Geometry check sheet. Reference: the model listing, model coordinates, mm. A direction names the side the tool comes from. Coordinates: 2 decimals unless noted, no trailing zeros. Write each loop counter-clockwise with the first axis right and the second up, starting at its lowest first coordinate (ties: lowest second). Pieces come first, ordered by that corner, then holes. Notation, with made-up numbers: (-5.5, 80.5) -> (52.5, 80.5) arc R15 cw to (52.5, 98.5) -> close; hole circle Ø1 at (35.5, 83.25). An arc over 180 degrees is marked (long way). Answer as CSV lines item,"result".
```python
from build123d import *

# Parameters (mm, degrees)
EXTRUDE_THIN1_DEPTH     = 60
CUT_EXTRUDE1_DEPTH      = 1
CUT_EXTRUDE1_DEPTH_BACK = 47


with BuildPart() as part:
    # Sketch1 → Extrude-Thin1 (new body, symmetric)
    with BuildSketch(Plane.XY):
        with BuildLine():
            Line((-33, 15), (-33, -15))
            ThreePointArc((-33, -15), (-30.656854249, -20.656854249), (-25, -23))
            Line((-25, -23), (25, -23))
            ThreePointArc((25, -23), (30.656854249, -20.656854249), (33, -15))
            Line((33, -15), (33, 15))
            ThreePointArc((33, 15), (30.656854249, 20.656854249), (25, 23))
            Line((25, 23), (-25, 23))
            ThreePointArc((-25, 23), (-30.656854249, 20.656854249), (-33, 15))
        make_face()
        with BuildLine():
            Line((-30, 15), (-30, -15))
            ThreePointArc((-30, -15), (-28.535533906, -18.535533906), (-25, -20))
            Line((-25, -20), (25, -20))
            ThreePointArc((25, -20), (28.535533906, -18.535533906), (30, -15))
            Line((30, -15), (30, 15))
            ThreePointArc((30, 15), (28.535533906, 18.535533906), (25, 20))
            Line((25, 20), (-25, 20))
            ThreePointArc((-25, 20), (-28.535533906, 18.535533906), (-30, 15))
        make_face(mode=Mode.SUBTRACT)
    extrude(amount=EXTRUDE_THIN1_DEPTH, both=True)

    # Sketch2 → Cut-Extrude1 (cut, two sides)
    with BuildSketch(Plane(origin=(0, 23, 0), x_dir=(1, 0, 0), z_dir=(0, 1, 0))) as cut_extrude1_sk:
        with BuildLine():
            Line((6, 45), (6, -45))
            ThreePointArc((6, -45), (0, -51), (-6, -45))
            Line((-6, -45), (-6, 45))
            ThreePointArc((-6, 45), (0, 51), (6, 45))
        make_face()
    extrude(amount=CUT_EXTRUDE1_DEPTH, mode=Mode.SUBTRACT)
    extrude(cut_extrude1_sk.sketch, amount=-CUT_EXTRUDE1_DEPTH_BACK, mode=Mode.SUBTRACT)


solid = part.part
```
Item 1: Cross-section at C-C, the plane x = 0. Record the cut outline in (y, z).
Responses:
outline,"(-23, -60) -> (-20, -60) -> (-20, -51) -> (-23, -51) -> close; (-23, 51) -> (-20, 51) -> (-20, 60) -> (-23, 60) -> close; (20, -60) -> (23, -60) -> (23, -51) -> (20, -51) -> close; (20, 51) -> (23, 51) -> (23, 60) -> (20, 60) -> close"
Item 2: Release check for a two-part mould opening along Z. For faces 4 (the flat face through (-11, -20, 1)), 5 (the cylindrical face through (0, -21, 51)), 6 (the flat face through (-6, -21, 1)), 7 (the flat face through (0, 21, 60)) record: +Z half, -Z half, draft (parallel to the pull), parting line (faces both ways), or undercut.
Responses:
face 4,"draft"
face 5,"undercut"
face 6,"undercut"
face 7,"+Z half"
Item 3: Thickness scan on probe 1 along Y at (x, z) = (-8.5, -15.5); probe 2 along X at (y, z) = (8, -33); probe 3 along X at (y, z) = (-18, 33). Record the ranges inside material, lowest first.
Responses:
probe 1,"y = -23 to -20, 20 to 23"
probe 2,"x = -33 to -30, 30 to 33"
probe 3,"x = -32.42 to -29, 29 to 32.42"
Item 4: Depth check by flat-ended pin: pin 1 Ø0.9 at (y, z) = (22, -18) entering from +X; pin 2 Ø2.5 at (y, z) = (21, 14) entering from -X; pin 3 Ø6 at (x, y) = (23, -15) entering from -Z; pin 4 Ø2.5 at (y, z) = (-21.5, 1) entering from -X. Enter the tip coordinate at first touch or a pass-through.
Responses:
pin 1,"stops at x = 29.59"
pin 2,"stops at x = -31.44"
pin 3,"passes through"
pin 4,"stops at x = -31.04"
Item 5: Set-up check for faces 1 (the cylindrical face through (0, -21, -51)), 2 (the flat face through (33, 0, 1)), 3 (the flat face through (30, 0, 1)): record each of +Z, -Z, +X, -X, +Y, -Y from which the full face is reachable in a straight line by a thin tool's end or side.
Responses:
face 1,"+Y, -Y"
face 2,"+Z, -Z, +X, +Y, -Y"
face 3,"+Z, -Z"
Item 6: Cross-section at A-A, the plane z = -18.5. Record the cut outline in (x, y).
Responses:
outline,"(-33, -15) arc R8 ccw to (-25, -23) -> (-6, -23) -> (-6, -20) -> (-25, -20) arc R5 cw to (-30, -15) -> (-30, 15) arc R5 cw to (-25, 20) -> (-6, 20) -> (-6, 23) -> (-25, 23) arc R8 ccw to (-33, 15) -> close; (6, -23) -> (25, -23) arc R8 ccw to (33, -15) -> (33, 15) arc R8 ccw to (25, 23) -> (6, 23) -> (6, 20) -> (25, 20) arc R5 cw to (30, 15) -> (30, -15) arc R5 cw to (25, -20) -> (6, -20) -> close"
Item 7: Cross-section at B-B, the plane y = 0. Record the cut outline in (x, z).
Responses:
outline,"(-33, -60) -> (-30, -60) -> (-30, 60) -> (-33, 60) -> close; (30, -60) -> (33, -60) -> (33, 60) -> (30, 60) -> close"
Item 8: Cross-section at D-D, the plane x = -15.5. Record the cut outline in (y, z).
Responses:
outline,"(-23, -60) -> (-20, -60) -> (-20, 60) -> (-23, 60) -> close; (20, -60) -> (23, -60) -> (23, 60) -> (20, 60) -> close"
